The listing builds one solid part. Answer for the finished solid, in the listing's coordinates (mm). Coordinates: 2 decimals unless noted, no trailing zeros. Order: outer loops, then holes, each group sorted by start corner. A loop starts at its lowest first (then second) coordinate and runs counter-clockwise, first axis right, second up. Notation, with made-up numbers: (52.5, -30.5) -> (101.5, -30.5) arc R17 ccw to (101.5, -17.5) -> close; hole circle Ø8 at (62, 47.25). An arc over 180 degrees is marked (long way). Return JSON: item names as keys, results as strings.
```python
from build123d import *

# Parameters (mm, degrees)
F0_W     = 28
F0_H     = 40
F0_R     = 1.6
F0_W_2   = 10
F0_H_2   = 35
F1_DEPTH = 3
F2_SIZE  = 5
F3_SIZE  = 3
F4_SIZE  = 7


with BuildPart() as f1:
    # F0 (on Top) → F1 (new body)
    with BuildSketch(Plane.XY):
        with Locations((0, 80)):
            Rectangle(F0_W, F0_H)
        with Locations((-9, 95)):
            Circle(F0_R, mode=Mode.SUBTRACT)
        with Locations((9, 95)):
            Circle(F0_R, mode=Mode.SUBTRACT)
        with Locations((19, 42.5)):
            Rectangle(F0_W_2, F0_H_2)
        with BuildLine():
            ThreePointArc((17.4, 55), (19, 56.6), (20.6, 55))
            Line((20.6, 55), (20.6, 30))
            ThreePointArc((20.6, 30), (19, 28.4), (17.4, 30))
            Line((17.4, 30), (17.4, 55))
        make_face(mode=Mode.SUBTRACT)
        with BuildLine():
            Line((14, 25), (14, 60))
            Line((14, 60), (-14, 60))
            Line((-14, 60), (-14, 25))
            Line((-14, 25), (-1.6, 25))
            Line((-1.6, 25), (-1.6, 45))
            ThreePointArc((-1.6, 45), (0, 46.6), (1.6, 45))
            Line((1.6, 45), (1.6, 25))
            Line((1.6, 25), (14, 25))
        make_face()
        with Locations((-19, 42.5)):
            Rectangle(F0_W_2, F0_H_2)
        with BuildLine():
            ThreePointArc((-20.6, 55), (-19, 56.6), (-17.4, 55))
            Line((-17.4, 55), (-17.4, 30))
            ThreePointArc((-17.4, 30), (-19, 28.4), (-20.6, 30))
            Line((-20.6, 30), (-20.6, 55))
        make_face(mode=Mode.SUBTRACT)
        with BuildLine():
            Line((14, -100), (14, 25))
            Line((14, 25), (1.6, 25))
            Line((1.6, 25), (1.6, 20))
            ThreePointArc((1.6, 20), (0, 18.4), (-1.6, 20))
            Line((-1.6, 20), (-1.6, 25))
            Line((-1.6, 25), (-14, 25))
            Line((-14, 25), (-14, -100))
            Line((-14, -100), (14, -100))
        make_face()
        with BuildLine():
            ThreePointArc((-10.6, -50), (-9, -48.4), (-7.4, -50))
            Line((-7.4, -50), (-7.4, -80))
            ThreePointArc((-7.4, -80), (-9, -81.6), (-10.6, -80))
            Line((-10.6, -80), (-10.6, -50))
        make_face(mode=Mode.SUBTRACT)
        with Locations((-9, -15)):
            Circle(F0_R, mode=Mode.SUBTRACT)
        with BuildLine():
            Line((1.6, -65), (1.6, -95))
            ThreePointArc((1.6, -95), (0, -96.6), (-1.6, -95))
            Line((-1.6, -95), (-1.6, -65))
            ThreePointArc((-1.6, -65), (0, -63.4), (1.6, -65))
        make_face(mode=Mode.SUBTRACT)
        with BuildLine():
            Line((10.6, -50), (10.6, -80))
            ThreePointArc((10.6, -80), (9, -81.6), (7.4, -80))
            Line((7.4, -80), (7.4, -50))
            ThreePointArc((7.4, -50), (9, -48.4), (10.6, -50))
        make_face(mode=Mode.SUBTRACT)
        with Locations((9, -15)):
            Circle(F0_R, mode=Mode.SUBTRACT)
    extrude(amount=F1_DEPTH)

    # F2
    f2_edges = [f1.edges().sort_by_distance(p)[0] for p in [
        (-14, 100, 1.5),
        (14, 100, 1.5),
        (-24, 60, 1.5),
        (24, 60, 1.5),
        (-24, 25, 1.5),
        (24, 25, 1.5),
    ]]
    chamfer(f2_edges, length=F2_SIZE)

    # F3
    f3_edges = [f1.edges().sort_by_distance(p)[0] for p in [
        (14, 25, 1.5),
        (-14, 25, 1.5),
        (-14, 60, 1.5),
        (14, 60, 1.5),
    ]]
    chamfer(f3_edges, length=F3_SIZE)

    # F4
    f4_edges = [f1.edges().sort_by_distance(p)[0] for p in [
        (14, -100, 1.5),
        (-14, -100, 1.5),
    ]]
    chamfer(f4_edges, length=F4_SIZE)


solid = f1.part
```
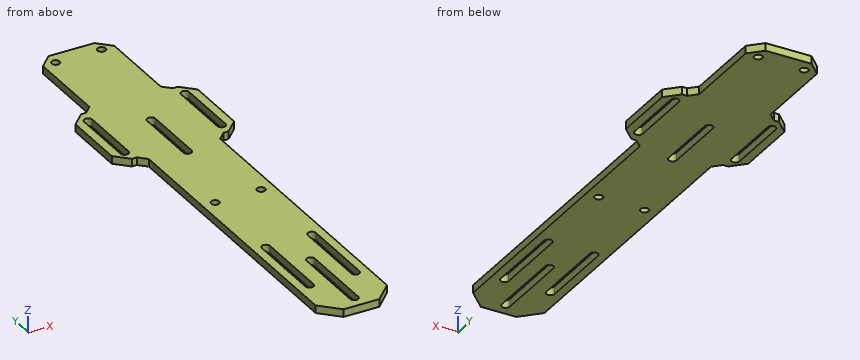
Item 1: The part is cut by section B-B on z = 1.55. Count the separate pieces of the cut face and the enclosed holes in it, plus the area to 3 significant figures.
Answer list:
{"separate pieces": "1", "enclosed holes": "10", "area": "5,590 mm2"}
Item 2: The part is cut by section C-C on y = -9. Determine the outline of the cut face in (x, z).
Answer list:
{"outline": "(-14, 0) -> (14, 0) -> (14, 3) -> (-14, 3) -> close"}
Item 3: Find the intervals of material crossed by probe 1 along X at (y, z) = (-59.5, 1.05); probe 2 along X at (y, z) = (53, 1.4); probe 3 along Y at (x, z) = (8, 2.1), in increasing order.
Answer list:
{"probe 1": "-14 to -10.6, -7.4 to 7.4, 10.6 to 14", "probe 2": "-24 to -20.6, -17.4 to 17.4, 20.6 to 24", "probe 3": "-99 to -81.25, -48.75 to -16.25, -13.75 to 93.75, 96.25 to 100"}
Item 4: Flat-ended cylindrical pins translate along their axes: pin 1 (0.9 mm diameter, centred on y = 75.5, z = 1, fed in from -X); pin 2 (3 mm diameter, centred on x = -9, y = -15, fed in from +Z); pin 3 (1.6 mm diameter, centred on x = -17.5, z = 1.5, fed in from -Y); pin 4 (1 mm diameter, centred on x = 18, z = 1, fed in from -Y). Find the tip coordinate at first contact, or state that the pin passes through.
Answer list:
{"pin 1": "x = -14", "pin 2": "through", "pin 3": "y = 24.7", "pin 4": "y = 25"}
Item 5: The part is cut by section A-A on y = -86. Determine the outline of the cut face in (x, z).
Answer list:
{"outline": "(-14, 0) -> (-1.6, 0) -> (-1.6, 3) -> (-14, 3) -> close; (1.6, 0) -> (14, 0) -> (14, 3) -> (1.6, 3) -> close"}
